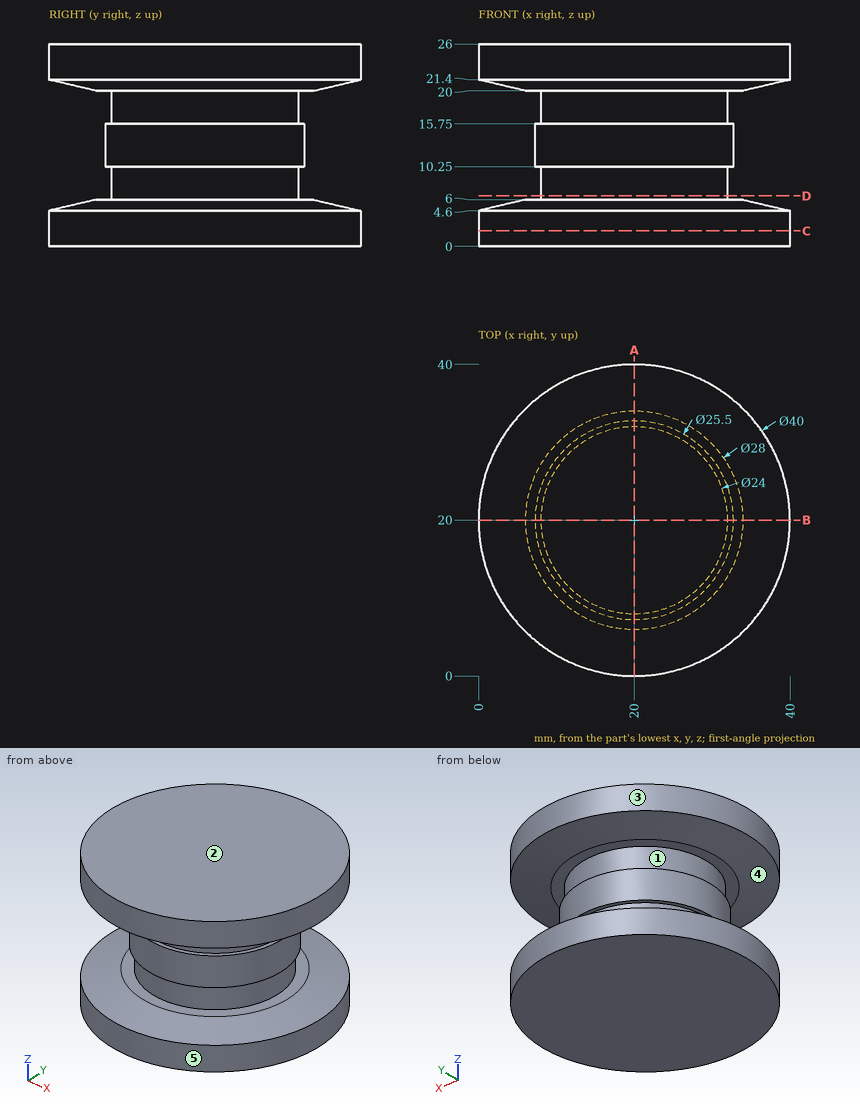
Can you work these out from the drawing? Everything is in mm from the part's minimum corner. A direction names the side the tool comes from. Coordinates: 2 decimals unless noted, no trailing zeros. Loops run counter-clockwise (first coordinate to the right, second up) from the corner with the lowest first, then second, coordinate; pieces in that order, holes last. Notation, with made-up numbers: (38, -13) -> (43, -13) arc R8 ccw to (43, 2) -> close; hole circle Ø1 at (22, 29). An arc over 180 degrees is marked (long way). Return JSON: item names as keys, results as strings.
1) For the marked faces 4 and 5, which set-ups out of +Z, -Z, +X, -X, +Y, -Y let a thin tool reach every point of the face, with its end or its side?
Results below:
{"face 4": "none", "face 5": "+Z, -Z"}
2) I need wall thicknesses on line 1 (Z direction, x = 30, y = 12.5); line 2 (Z direction, x = 34, y = 19); line 3 (Y direction, x = 20, z = 13.5). Which ranges of each line are inside material? Lowest first, please. Write a range as from..to.
Results below:
{"line 1": "0..6, 10.25..15.75, 20..26", "line 2": "0..5.99, 20.01..26", "line 3": "7.25..32.75"}
3) Thinking about a two-plate mould opening in Z: for the marked faces 1, 2 and 3, which applies, +Z half, -Z half, draft (parallel to the pull), parting line (faces both ways), or undercut?
Results below:
{"face 1": "undercut", "face 2": "+Z half", "face 3": "draft"}
4) If we section it at C-C, the plane z = 2: Write out the boundary of the cut face in (x, y).
Results below:
{"outline": "circle Ø40 at (20, 20)"}
5) If we section it at A-A, the plane x = 20: Write out the boundary of the cut face in (y, z), then the cut area to 3 significant figures.
Results below:
{"outline": "(0, 0) -> (40, 0) -> (40, 4.6) -> (34, 6) -> (32, 6) -> (32, 10.25) -> (32.75, 10.25) -> (32.75, 15.75) -> (32, 15.75) -> (32, 20) -> (34, 20) -> (40, 21.4) -> (40, 26) -> (0, 26) -> (0, 21.4) -> (6, 20) -> (8, 20) -> (8, 15.75) -> (7.25, 15.75) -> (7.25, 10.25) -> (8, 10.25) -> (8, 6) -> (6, 6) -> (0, 4.6) -> close", "area": "807 mm²"}
6) If we section it at D-D, the plane z = 6.5: Write out the boundary of the cut face in (x, y).
Results below:
{"outline": "circle Ø24 at (20, 20)"}
7) Will these pins go through, and if not, where does the flat tip stop? pin 1 (8 mm diameter, centred on x = 25, z = 20, fed in from -Y); pin 2 (6 mm diameter, centred on x = 23.5, z = 11.5, fed in from -Y); pin 3 (3 mm diameter, centred on x = 25.5, z = 5.5, fed in from -Y).
Results below:
{"pin 1": "y = 0.04", "pin 2": "y = 7.26", "pin 3": "y = 0.47"}
